Autodesk Inventor part; units mm, degrees
ref_plane "YZ Plane" through (0, 0, 0) normal (1, 0, 0) x (0, 1, 0)
ref_plane "XZ Plane" through (0, 0, 0) normal (0, 1, 0) x (-1, 0, 0)
ref_plane "XY Plane" through (0, 0, 0) normal (0, 0, 1) x (1, 0, 0)
sketch "Sketch1" plane through (0, 0, 0) normal (0, 1, 0) x (-1, 0, 0)
  line L0 (111.0745, 206.7031) -> (-41.3255, 206.7031)
  line L1 (-41.3255, 206.7031) -> (-41.3255, -364.7969)
  line L2 (-41.3255, -364.7969) -> (111.0745, -364.7969)
  line L3 (111.0745, -364.7969) -> (111.0745, 206.7031)
  point P0 (0, 0)
  dimension "d0" = 571.5
  dimension "d1" = 152.4
extrude "Extrusion1" add sketch "Sketch1" along normal blind 25.4
sketch "Sketch2" plane through (-111.0745, 0, 206.7031) normal (0, 0, 1) x (1, 0, 0)
  line L0 (0, 0) -> (0, 25.4)
  line L1 (0, 25.4) -> (152.4, 25.4)
  line L2 (152.4, 25.4) -> (152.4, -127)
  line L3 (152.4, -127) -> (0, -127)
  line L4 (0, -127) -> (0, 25.4)
  line L5 (152.4, 0) -> (152.4, 25.4)
  line L6 (0, 0) -> (152.4, 0)
  line L7 (0, -127) -> (152.4, -127)
  line L8 (152.4, -127) -> (152.4, -101.6)
  line L9 (152.4, -101.6) -> (0, -101.6)
  line L10 (0, -101.6) -> (0, -127)
  circle A0 centre (63.5, -101.6) radius 4.7625
  circle A1 centre (88.9, -101.6) radius 4.7625
  line L11 (0, -127) -> (63.5, -101.6) construction
  line L12 (88.9, -101.6) -> (152.4, -127) construction
  point P0 (111.0745, 0)
  point P1 (58.7375, -101.6)
  point P2 (68.2625, -101.6)
  point P3 (84.1375, -101.6)
  point P4 (93.6625, -101.6)
  dimension "d5" = 127
  dimension "d6" = 25.4
  dimension "d7" = 25.4
  dimension "d8" = 9.525
extrude "Extrusion2" add sketch "Sketch2" along normal blind 25.4 contours L6 L2 L9 A1 A0 L4 | L0 L1 L2 L6 | L9 A0 A1 L2 L3 L4
sketch "Sketch3" plane through (41.3255, 0, -364.7969) normal (0, 0, -1) x (-1, 0, 0)
  line L0 (0, 25.4) -> (152.4, 25.4)
  line L1 (152.4, 0) -> (152.4, -127)
  line L2 (0, 25.4) -> (152.4, 25.4)
  line L3 (152.4, 25.4) -> (152.4, -127)
  line L4 (152.4, -127) -> (0, -127)
  line L5 (0, -127) -> (0, 25.4)
  circle A0 centre (63.5, -101.6) radius 4.7625
  circle A1 centre (63.5, -101.6) radius 4.7625
  circle A2 centre (88.9, -101.6) radius 4.7625
  circle A3 centre (88.9, -101.6) radius 4.7625
  point P0 (41.3255, 0)
  dimension "d15" = 9.525
  dimension "d16" = 9.525
extrude "Extrusion3" add sketch "Sketch3" along normal blind 25.4
sketch "Sketch4" plane through (0, 25.4, 0) normal (0, 1, 0) x (1, 0, 0)
  line L0 (-52.337, 390.1969) -> (-42.812, 390.1969) construction
  line L1 (41.3255, -232.1031) -> (-111.0745, -232.1031) construction
  line L2 (-111.0745, -232.1031) -> (-111.0745, 390.1969) construction
  line L3 (-111.0745, 79.0469) -> (41.3255, 79.0469) construction
  line L4 (41.3255, 390.1969) -> (41.3255, -232.1031) construction
  line L5 (41.3255, 390.1969) -> (-111.0745, 390.1969) construction
  circle A0 centre (-60.2745, 79.0469) radius 12.7
  point P0 (0, 0)
  dimension "d17" = 25.4
  dimension "d20" = 50.8
extrude "Extrusion4" cut sketch "Sketch4" against normal through all
sketch "Sketch5" plane through (0, 25.4, 0) normal (0, 1, 0) x (1, 0, 0)
  line L0 (-111.0745, -232.1031) -> (-111.0745, 390.1969)
  line L1 (-111.0745, 282.2469) -> (-619.0745, 282.2469)
  line L2 (-619.0745, 282.2469) -> (-619.0745, -124.1531)
  line L3 (-619.0745, -124.1531) -> (-111.0745, -124.1531)
  line L4 (-111.0745, -124.1531) -> (-111.0745, 282.2469)
  line L5 (41.3255, 390.1969) -> (-111.0745, 390.1969) construction
  line L6 (-619.0745, 282.2469) -> (-111.0745, 390.1969) construction
  line L7 (-111.0745, -232.1031) -> (-619.0745, -124.1531) construction
  point P0 (0, 0)
  point P1 (-111.0745, -124.1531)
  dimension "d21" = 508
  dimension "d22" = 406.4
extrude "Extrusion5" add sketch "Sketch5" against normal blind 25.4
sketch "Sketch6" plane through (0, 25.4, 0) normal (0, 1, 0) x (1, 0, 0)
  line L0 (-619.0745, -124.1531) -> (-619.0745, 282.2469) construction
  line L1 (-619.0745, 282.2469) -> (-441.2745, 282.2469) construction
  line L2 (-441.2745, 282.2469) -> (-441.2745, -124.1531) construction
  line L3 (-441.2745, -124.1531) -> (-619.0745, -124.1531) construction
  line L4 (-619.0745, -124.1531) -> (-619.0745, 282.2469) construction
  circle A0 centre (-441.2745, 212.3969) radius 3.175
  circle A1 centre (-441.2745, -54.3031) radius 3.175
  line L5 (-619.0745, -124.1531) -> (-111.0745, -124.1531)
  line L6 (-111.0745, 282.2469) -> (-619.0745, 282.2469)
  line L7 (-111.0745, -232.1031) -> (-111.0745, -124.1531)
  line L8 (-111.0745, 282.2469) -> (-111.0745, 390.1969)
  point P0 (0, 0)
  dimension "d26" = 69.85
  dimension "d27" = 69.85
  dimension "d28" = 6.35
  dimension "d33" = 330.2
  dimension "d34" = 330.2
extrude "Extrusion6" cut sketch "Sketch6" against normal through all
sketch "Sketch7" plane through (0, 25.4, 0) normal (0, 1, 0) x (1, 0, 0)
  line L0 (41.3255, -206.7031) -> (41.3255, 364.7969) construction
  line L1 (41.3255, 364.7969) -> (-365.0745, 364.7969) construction
  line L2 (-365.0745, 364.7969) -> (-365.0745, -206.7031) construction
  line L3 (-365.0745, -206.7031) -> (41.3255, -206.7031) construction
  line L4 (41.3255, -206.7031) -> (41.3255, 364.7969) construction
  line L5 (-619.0745, 282.2469) -> (-111.0745, 282.2469) construction
  line L6 (-365.0745, 282.2469) -> (-415.8745, 282.2469) construction
  line L7 (-415.8745, 282.2469) -> (-415.8745, -124.1531) construction
  line L8 (-415.8745, -124.1531) -> (-365.0745, -124.1531) construction
  line L9 (-365.0745, -124.1531) -> (-365.0745, 282.2469) construction
  line L10 (-415.8745, 282.2469) -> (-365.0745, 282.2469) construction
  line L11 (-365.0745, 282.2469) -> (-365.0745, -124.1531) construction
  line L12 (-365.0745, -124.1531) -> (-415.8745, -124.1531) construction
  line L13 (-415.8745, -124.1531) -> (-415.8745, 282.2469) construction
  line L14 (-415.8745, 206.0469) -> (-365.0745, 206.0469)
  line L15 (-365.0745, 206.0469) -> (-365.0745, 155.2469)
  line L16 (-365.0745, 155.2469) -> (-415.8745, 155.2469)
  line L17 (-415.8745, 155.2469) -> (-415.8745, 206.0469)
  line L18 (-415.8745, -47.9531) -> (-365.0745, -47.9531)
  line L19 (-365.0745, -47.9531) -> (-365.0745, 2.8469)
  line L20 (-365.0745, 2.8469) -> (-415.8745, 2.8469)
  line L21 (-415.8745, 2.8469) -> (-415.8745, -47.9531)
  point P0 (0, 0)
  dimension "d31" = 406.4
  dimension "d35" = 406.4
  dimension "d36" = 50.8
  dimension "d39" = 152.4
  dimension "d40" = 50.8
  dimension "d41" = 50.8
  dimension "d42" = 76.2
  dimension "d43" = 76.2
extrude "Extrusion7" add sketch "Sketch7" along normal blind 50.8
sketch "Sketch9" plane through (-415.8745, 25.4, 47.9531) normal (0, 0, 1) x (1, 0, 0)
  line L0 (50.8, 0) -> (50.8, 50.8) construction
  line L1 (50.8, 50.8) -> (0, 50.8) construction
  line L2 (50.8, 25.4) -> (25.4, 25.4) construction
  line L3 (25.4, 25.4) -> (25.4, 50.8) construction
  line L4 (25.4, 50.8) -> (50.8, 50.8) construction
  line L5 (50.8, 50.8) -> (50.8, 25.4) construction
  circle A0 centre (25.4, 25.4) radius 12.7
  point P0 (415.8745, -25.4)
  dimension "d44" = 25.4
extrude "Extrusion8" cut sketch "Sketch9" against normal through all
fillet "Fillet1" radius 25.4 4 edges at (-415.8745, 76.2, 22.5531) (-365.0745, 76.2, 22.5531) (-415.8745, 76.2, -180.6469) (-365.0745, 76.2, -180.6469)
equation "\"d27\" = d26"
equation "\"BendRadius\" = Thickness"
equation "\"BendReliefWidth\" = Thickness"
equation "\"BendReliefDepth\" = 0.5 * Thickness"
equation "\"CornerReliefSize\" = 4 * Thickness"
equation "\"MinimumRemnant\" = 2 * Thickness"
equation "\"TransitionRadius\" = BendRadius"
equation "\"JacobiRadiusSize\" = BendRadius"
equation "\"GapSize\" = Thickness"
properties part number "Steering Mount"
The model under review builds one solid part; all positions refer to its coordinate system, in mm. A direction names the side the tool comes from. Give positions to 0.01 mm unless a question says otherwise; leave off trailing zeros. Write each loop counter-clockwise with the first axis right and the second up, starting at its lowest first coordinate (ties: lowest second). Pieces come first, ordered by that corner, then holes. Notation, with made-up numbers: M 89,-9.5 L 125,-9.5 A20 cw 125,23.5 Z; hole C 23,31.5 d1. An arc over 180 degrees is marked long. Answer in a Markdown table with one row per item.
Item 1: Add section A-A on x = -7.5. Give the boundary of the cut face in (y, z), plus the area to 3 significant figures.
Check sheet entries:
| item | result |
|---|---|
| outline | M -127,-390.2 L 25.4,-390.2 L 25.4,232.1 L -127,232.1 L -127,206.7 L 0,206.7 L 0,-364.8 L -127,-364.8 Z |
| area | 22,300 mm2 |
Item 2: Draft analysis for pull direction X (two halves, no side actions). For faces 1 (the face through (-34, -127, 219)), 2 (the face through (-378.36, 54.61, 22.91)), 3 (the face through (-408.631, 68.562, -181.002)), state which applies: +X half, -X half, draft (parallel to the pull), parting line (faces both ways), or undercut.
Check sheet entries:
| item | result |
|---|---|
| face 1 | draft |
| face 2 | undercut |
| face 3 | -X half |
Item 3: Add section C-C on x = -489.5. Give the boundary of the cut face in (y, z), plus the area to 3 significant figures.
Check sheet entries:
| item | result |
|---|---|
| outline | M 0,-282.25 L 25.4,-282.25 L 25.4,124.15 L 0,124.15 Z |
| area | 10,300 mm2 |
Item 4: Add section B-B on z = -351.5. Give the boundary of the cut face in (x, y).
Check sheet entries:
| item | result |
|---|---|
| outline | M -111.07,0 L 41.33,0 L 41.33,25.4 L -111.07,25.4 Z |
Item 5: Tool access review of faces 4 (the face through (-111.074, -16, -371)), 5 (the face through (-384, 39, -2.847)), 6 (the face through (-36, -63, 206.703)), 7 (the face through (-415.874, 38, -180)): name each direction out of +Z, -Z, +X, -X, +Y, -Y from which nothing blocks a thin tool from reaching the whole face with its end or side.
Check sheet entries:
| item | result |
|---|---|
| face 4 | -Z, -X, +Y, -Y |
| face 5 | +X, -X, +Y |
| face 6 | +X, -X, -Y |
| face 7 | +Z, -Z, -X, +Y |
Item 6: For line 1 along X through (y, z) = (-101, 218); line 2 along X through (y, z) = (-101.6, 212.5); line 3 along Z through (x, y) = (-17.5, -59), list the stretches that pass through material, from the lowest coordinate up.
Check sheet entries:
| item | result |
|---|---|
| line 1 | -111.07 to -52.3, -42.85 to -26.9, -17.45 to 41.33 |
| line 2 | -111.07 to -52.34, -42.81 to -26.94, -17.41 to 41.33 |
| line 3 | -390.2 to -364.8, 206.7 to 232.1 |
Item 7: For P1, Ø12.5, axis at y = 39.5, z = -177.5, coming from the +X side; P2, Ø20.5, axis at x = -257.5, y = 19, coming from the -Z side; P3, Ø1.5, axis at x = -492.5, z = -80, coming from the -Y side; P4, Ø5.5, axis at x = -47.57, y = -101.6, coming from the -Z side, all flat-tipped, find the tip position at first contact; note any pin that passes through.
Check sheet entries:
| item | result |
|---|---|
| P1 | x = -365.07 |
| P2 | z = -282.25 |
| P3 | y = 0 |
| P4 | through |
